```python
from build123d import *

# Parameters (mm, degrees)
BASIS_LINEAR_AUSTRAGEN_DEPTH = 8
BOHRUNG1_D                   = 14


with BuildPart() as part:
    # Skizze1 → Basis-Linear austragen (new body)
    with BuildSketch(Plane.XY):
        Polygon((0, -13.856406461), (12, -6.92820323), (12, 6.92820323), (0, 13.856406461), (-12, 6.92820323), (-12, -6.92820323), align=None)
    extrude(amount=BASIS_LINEAR_AUSTRAGEN_DEPTH)

    # Skizze2 → Schnitt-Rotation1 (revolve, cut)
    with BuildSketch(Plane(origin=(0, 0, 0), x_dir=(0, 0, -1), z_dir=(1, 0, 0))):
        Polygon((-8, 12), (-6.92820323, 13.856406461), (-1.07179677, 13.856406461), (0, 12), (0, 14.856406461), (-8, 14.856406461), align=None)
    revolve(axis=Axis((0, 0, -0.921105868), (0, 0, 1)), mode=Mode.SUBTRACT)

    # Bohrung1 (through all)
    with Locations(Plane.XY.offset(8)):
        with Locations((0, 0)):
            Hole(BOHRUNG1_D / 2)


solid = part.part
```
Build history of the part. All positions in model axes, mm. Round coordinates to 2 decimals unless told otherwise and drop trailing zeros. Write each loop counter-clockwise with the first axis right and the second up, starting at its lowest first coordinate (ties: lowest second). Pieces come first, ordered by that corner, then holes. Notation, with made-up numbers: (74.25, -19) - (90.25, -19) arc R29 ccw to (90.25, 13) - close; hole circle Ø8 at (48, 78.25). An arc over 180 degrees is marked (long way). Write each question's results on one line, items separated by ' | '. Start each with the question number.
Item 1: Drop flat-ended pins along their axis: P1, Ø3, axis at y = -8.5, z = 1.5, coming from the -X side; P2, Ø3, axis at y = 9.5, z = 1, coming from the +X side. Give the stop position or say it passes through.
Item 2: Mould opens along X. For faces 1 (the face through (10.76, -6.248, 0.256)), 2 (the face through (-6.466, -2.681, 3.944)), 3 (the face through (-5.92, 10.44, 3.94)), 4 (the face through (0.03, 12.45, 7.74)) say: pulls with the +X half, pulls with the -X half, needs draft (parallel to the pull), parting line crosses it, or undercut.
Item 3: Saw through at A-A (z = 2.75). Write the cut outline in (x, y).
Item 4: Saw through at B-B (z = 7.25). Write the cut outline in (x, y), and give its area (3 significant figures).
Item 5: Wall check: L1, parallel to Y at x = 4.75, z = 1.75; L2, parallel to X at y = 2, z = 3.25; L3, parallel to X at y = -5.5, z = 4.75. Give the ranges that are in metal, low to high. Write a range as [from, to].
Results are:
1) P1: stops at x = -11.88 | P2: stops at x = 10.14
2) face 1: pulls with the +X half | face 2: undercut | face 3: pulls with the -X half | face 4: parting line crosses it
3) outline: (-12, -6.93) - (0, -13.86) - (12, -6.93) - (12, 6.93) - (0, 13.86) - (-12, 6.93) - close; hole circle Ø14 at (0, 0)
4) outline: (-12, -5.73) arc R13.3 ccw to (-10.96, -7.53) - (-1.04, -13.26) arc R13.3 ccw to (1.04, -13.26) - (10.96, -7.53) arc R13.3 ccw to (12, -5.73) - (12, 5.73) arc R13.3 ccw to (10.96, 7.53) - (1.04, 13.26) arc R13.3 ccw to (-1.04, 13.26) - (-10.96, 7.53) arc R13.3 ccw to (-12, 5.73) - close; hole circle Ø14 at (0, 0) | area: 342 mm²
5) L1: y = [-11.11, -5.14], [5.14, 11.11] | L2: x = [-12, -6.71], [6.71, 12] | L3: x = [-12, -4.33], [4.33, 12]
